Build history of the part. All positions in model axes, mm. Face numbers are marked on the shaded views. Coordinates: 2 decimals unless noted, no trailing zeros. Order: outer loops, then holes, each group sorted by start corner. A loop starts at its lowest first (then second) coordinate and runs counter-clockwise, first axis right, second up. Notation, with made-up numbers: M 19.5,37.25 L 74.5,37.25 A27 cw 74.5,53.25 Z; hole C -19,51.25 d1. An arc over 180 degrees is marked long. Write item = value, one per line. Start each with the question number.
Q1. Drill centre lines: probe 1 along Y at (x, z) = (1.35, 2); probe 2 along X at (y, z) = (25, -0.6); probe 3 along X at (y, z) = (26, -0.2). Where is each one in solid material? Low to high.
Q2. Band-saw the part on D-D on y = 11.5. Write the cut outline in (x, z), plus the area to 3 significant figures.
Q3. Band-saw the part on C-C on x = -1.3. Write the cut outline in (y, z), plus the area to 3 significant figures.
Q4. Pull direction X, two halves, no side cores. Call the marked faces 1, 2 and 3: released by +X, released by -X, zero draft, split by the parting line, or undercut.
Q5. Pin check, flat tips, straight feed: P1, Ø2, axis at x = -2, y = 16, coming from the -Z side; P2, Ø2, axis at x = 0, y = 38, coming from the +Z side. Stop position of each tip, or through.
Q6. Band-saw the part on B-B on y = 38.5. Write the cut outline in (x, z).
Q7. Band-saw the part on A-A on z = 0. Write the cut outline in (x, y), plus the area to 3 significant figures.
```python
from build123d import *

# Parameters (mm, degrees)
SKETCH1_R           = 3
BOSS_EXTRUDE1_DEPTH = 20
SKETCH2_R           = 0.9
BOSS_EXTRUDE2_DEPTH = 13
SKETCH3_R           = 0.5
BOSS_EXTRUDE3_DEPTH = 15


with BuildPart() as part:
    # Sketch1 → Boss-Extrude1 (new body)
    with BuildSketch(Plane(origin=(0, 0, 0), x_dir=(1, 0, 0), z_dir=(0, 1, 0))):
        Circle(SKETCH1_R)
    extrude(amount=BOSS_EXTRUDE1_DEPTH)

    # Sketch2 → Boss-Extrude2 (add)
    with BuildSketch(Plane(origin=(0, 20, 0), x_dir=(1, 0, 0), z_dir=(0, 1, 0))):
        with Locations((1.27, 0)):
            Circle(SKETCH2_R)
        with Locations((-1.27, 0)):
            Circle(SKETCH2_R)
    extrude(amount=BOSS_EXTRUDE2_DEPTH)

    # Sketch3 → Boss-Extrude3 (add)
    with BuildSketch(Plane(origin=(0, 33, 0), x_dir=(1, 0, 0), z_dir=(0, 1, 0))):
        with Locations((1.27, 0)):
            Circle(SKETCH3_R)
        with Locations((-1.27, 0)):
            Circle(SKETCH3_R)
    extrude(amount=BOSS_EXTRUDE3_DEPTH)


solid = part.part
```
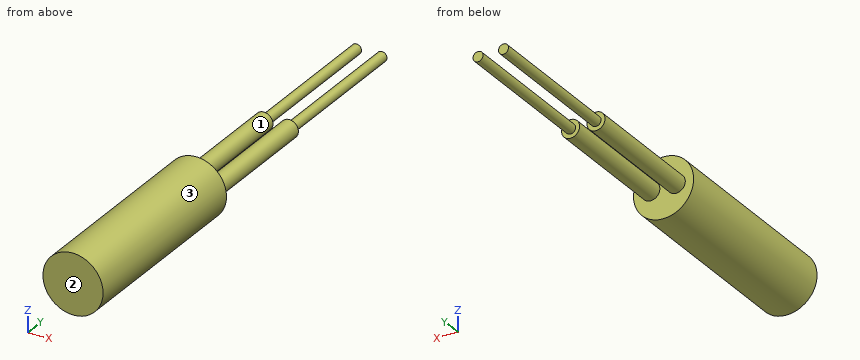
Recorded:
q1.probe_1 = 0 to 20
q1.probe_2 = -1.94 to -0.6, 0.6 to 1.94
q1.probe_3 = -2.15 to -0.39, 0.39 to 2.15
q2.outline = C 0,0 d6
q2.area = 28.3 mm2
q3.outline = M 0,-2.7 L 20,-2.7 L 20,-0.9 L 33,-0.9 L 33,-0.5 L 48,-0.5 L 48,0.5 L 33,0.5 L 33,0.9 L 20,0.9 L 20,2.7 L 0,2.7 Z
q3.area = 147 mm2
q4.face_1 = undercut
q4.face_2 = zero draft
q4.face_3 = split by the parting line
q5.P1 = -2.83
q5.P2 = 0.42
q6.outline = C -1.27,0 d1; C 1.27,0 d1
q7.outline = M -3,0 L 3,0 L 3,20 L 2.17,20 L 2.17,33 L 1.77,33 L 1.77,48 L 0.77,48 L 0.77,33 L 0.37,33 L 0.37,20 L -0.37,20 L -0.37,33 L -0.77,33 L -0.77,48 L -1.77,48 L -1.77,33 L -2.17,33 L -2.17,20 L -3,20 Z
q7.area = 197 mm2
